from build123d import *

# Parameters (mm, degrees)
BOSS_EXTRUDE1_DEPTH = 50
FILLET1_RADIUS      = 25
FILLET1_LENGTH      = 5
FILLET2_RADIUS      = 25
FILLET2_LENGTH      = 5
SKETCH2_W           = 111
SKETCH2_H           = 100
BOSS_EXTRUDE2_DEPTH = 5
SKETCH3_R           = 1.75
CUT_EXTRUDE1_DEPTH  = 204.28770253
SKETCH4_R           = 5
CUT_EXTRUDE2_DEPTH  = 256.203624582


with BuildPart() as part:
    # Sketch1 → Boss-Extrude1 (new body)
    with BuildSketch(Plane(origin=(0, 0, 0), x_dir=(1, 0, 0), z_dir=(0, 1, 0))):
        Polygon((0, 0), (0, 176.7), (101, 176.7), (101, 0), (53, 0), (53, -5), (53, -45), (58, -45), (58, -5), (106, -5), (106, 181.7), (-5, 181.7), (-5, -5), (43, -5), (43, -45), (48, -45), (48, -5), (48, 0), align=None)
    extrude(amount=BOSS_EXTRUDE1_DEPTH)

    # Fillet1: full round fillet: the end face becomes a half cylinder, R = half its width
    fillet1_face = Plane((45.5, 25, 45), x_dir=(1, 0, 0), z_dir=(0, 0, 1))  # on the end face: x along it, z out of the body
    fillet1_slab = fillet1_face.offset(-FILLET1_RADIUS / 2) * Box(FILLET1_LENGTH, 2 * FILLET1_RADIUS, FILLET1_RADIUS, mode=Mode.PRIVATE)  # the body's end, R deep
    fillet1_round = Plane((45.5, 25, 20), x_dir=(0, 0, 1), z_dir=(1, 0, 0)) * Cylinder(FILLET1_RADIUS, FILLET1_LENGTH, mode=Mode.PRIVATE)  # its axis R under the face
    add(fillet1_slab - fillet1_round, mode=Mode.SUBTRACT)

    # Fillet2: full round fillet: the end face becomes a half cylinder, R = half its width
    fillet2_face = Plane((55.5, 25, 45), x_dir=(1, 0, 0), z_dir=(0, 0, 1))  # on the end face: x along it, z out of the body
    fillet2_slab = fillet2_face.offset(-FILLET2_RADIUS / 2) * Box(FILLET2_LENGTH, 2 * FILLET2_RADIUS, FILLET2_RADIUS, mode=Mode.PRIVATE)  # the body's end, R deep
    fillet2_round = Plane((55.5, 25, 20), x_dir=(0, 0, 1), z_dir=(1, 0, 0)) * Cylinder(FILLET2_RADIUS, FILLET2_LENGTH, mode=Mode.PRIVATE)  # its axis R under the face
    add(fillet2_slab - fillet2_round, mode=Mode.SUBTRACT)

    # Sketch2 → Boss-Extrude2 (add)
    with BuildSketch(Plane(origin=(0, 0, -181.7), x_dir=(-1, 0, 0), z_dir=(0, 0, -1))):
        with Locations((-50.5, 0)):
            Rectangle(SKETCH2_W, SKETCH2_H)
    extrude(amount=BOSS_EXTRUDE2_DEPTH)

    # Sketch3 → Cut-Extrude1 (cut, through all)
    with BuildSketch(Plane.ZY.offset(-43)):
        with Locations((30, 25)):
            Circle(SKETCH3_R)
    extrude(amount=-CUT_EXTRUDE1_DEPTH, mode=Mode.SUBTRACT)

    # Sketch4 → Cut-Extrude2 (cut, through all)
    with BuildSketch(Plane.XY.offset(-181.7)):
        with Locations((50.5, -30)):
            Circle(SKETCH4_R)
    extrude(amount=-CUT_EXTRUDE2_DEPTH, mode=Mode.SUBTRACT)


solid = part.part
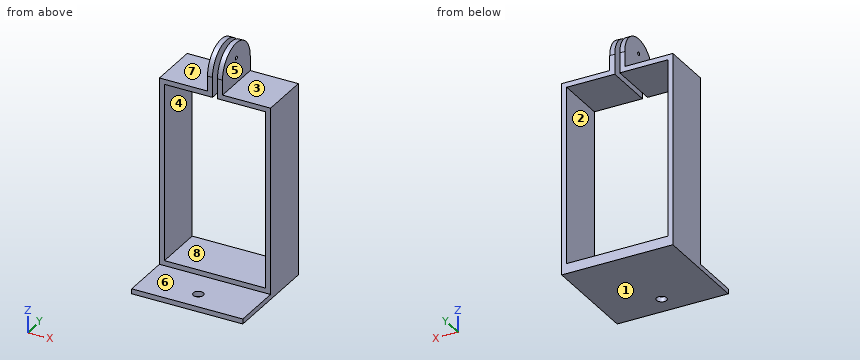
CAD build for the part. Positions are in the model's coordinates, mm. Face numbers are marked on the shaded views. A direction names the side the tool comes from. Coordinates: 2 decimals unless noted, no trailing zeros. Order: outer loops, then holes, each group sorted by start corner. A loop starts at its lowest first (then second) coordinate and runs counter-clockwise, first axis right, second up. Notation, with made-up numbers: (-40, 71) -> (-31, 71) arc R29 ccw to (-31, 93) -> close; hole circle Ø7 at (-38.75, 53.25). An arc over 180 degrees is marked (long way). Answer in a Markdown table with one row per item.
1) Mould opens along Z. For the marked faces 1, 2, 3 and 4 say: pulls with the +Z half, pulls with the -Z half, needs draft (parallel to the pull), parting line crosses it, or undercut.
Check values:
| item | result |
|---|---|
| face 1 | pulls with the -Z half |
| face 2 | undercut |
| face 3 | pulls with the +Z half |
| face 4 | undercut |
2) Band-saw the part on A-A (z = -80). List the corners of the cut face in (x, y), and give its area (3 significant figures).
Check values:
| item | result |
|---|---|
| outline | (-5, 0) -> (0, 0) -> (0, 50) -> (-5, 50) -> close; (101, 0) -> (106, 0) -> (106, 50) -> (101, 50) -> close |
| area | 500 mm2 |
3) Drill centre lines: line 1 (X direction, y = 21, z = -161); line 2 (Y direction, x = 50.5, z = -182.75); line 3 (Z direction, x = 26, y = -28.5). Where is each one in solid material? Low to high.
Check values:
| item | result |
|---|---|
| line 1 | -5 to 0, 101 to 106 |
| line 2 | -50 to -35, -25 to 50 |
| line 3 | -186.7 to -181.7 |
4) Band-saw the part on D-D (y = 43.5). List the corners of the cut face in (x, z).
Check values:
| item | result |
|---|---|
| outline | (-5, -186.7) -> (106, -186.7) -> (106, 5) -> (58, 5) -> (58, 36.82) -> (53, 36.82) -> (53, 0) -> (101, 0) -> (101, -176.7) -> (0, -176.7) -> (0, 0) -> (48, 0) -> (48, 36.82) -> (43, 36.82) -> (43, 5) -> (-5, 5) -> close |
5) Band-saw the part on B-B (x = 22). List the corners of the cut face in (y, z).
Check values:
| item | result |
|---|---|
| outline | (-50, -186.7) -> (50, -186.7) -> (50, -176.7) -> (0, -176.7) -> (0, -181.7) -> (-50, -181.7) -> close; (0, 0) -> (50, 0) -> (50, 5) -> (0, 5) -> close |
6) Flat gauge pins, fed straight in: P1, Ø24, axis at x = 21.5, y = 14, coming from the +Z side; P2, Ø22.5, axis at y = 33, z = 18.5, coming from the -X side. Where does each tip first touch, or does it go through?
Check values:
| item | result |
|---|---|
| P1 | z = 5 |
| P2 | x = 43 |
7) Band-saw the part on C-C (y = -30). List the corners of the cut face in (x, z).
Check values:
| item | result |
|---|---|
| outline | (-5, -186.7) -> (45.5, -186.7) -> (45.5, -181.7) -> (-5, -181.7) -> close; (55.5, -186.7) -> (106, -186.7) -> (106, -181.7) -> (55.5, -181.7) -> close |
8) Which spindle directions (+Z, -Z, +X, -X, +Y, -Y) get a long thin tool onto all of the face, cutting with end or side? Do the marked faces 5, 6, 7 and 8. Say none if no direction does.
Check values:
| item | result |
|---|---|
| face 5 | +Z, +X, +Y, -Y |
| face 6 | +Z, +X, -X, -Y |
| face 7 | +Z, -X, +Y, -Y |
| face 8 | +Y, -Y |
